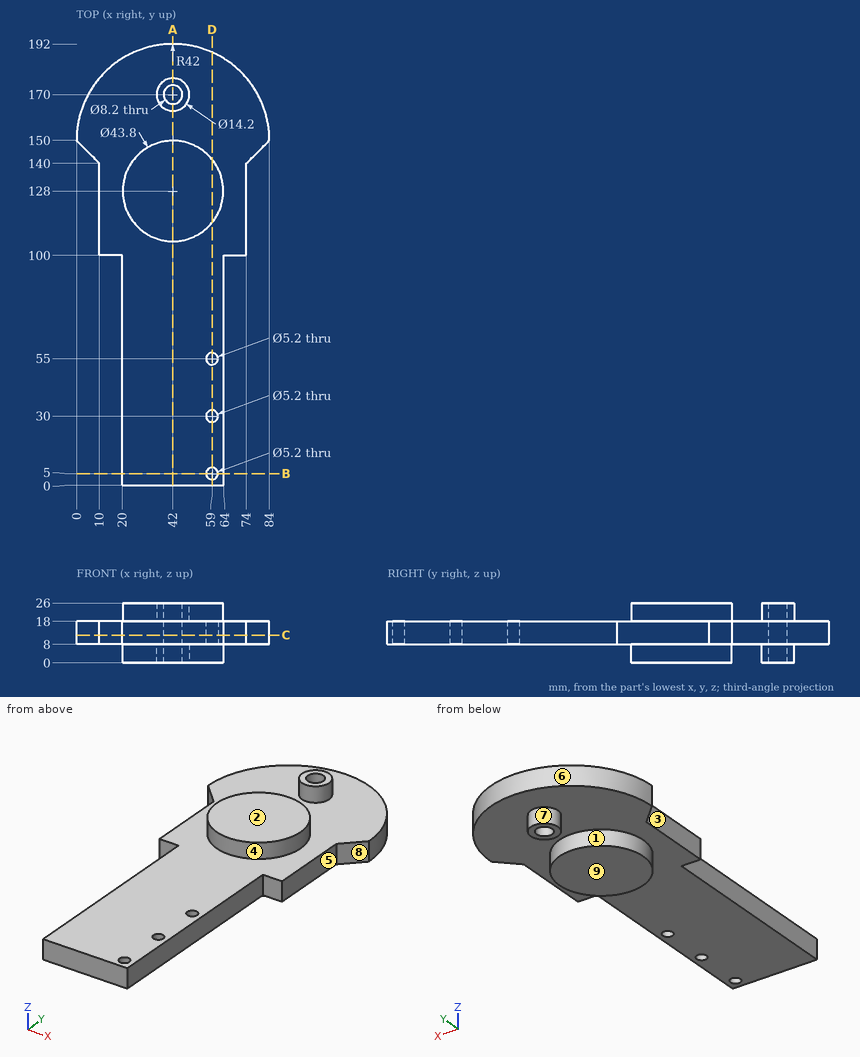
Check sheet for the drawn part. Datum: minimum x, y, z corner. Units: mm. A direction names the side the tool comes from. Round coordinates to 2 decimals unless told otherwise and drop trailing zeros. Order: outer loops, then holes, each group sorted by start corner. A loop starts at its lowest first (then second) coordinate and runs counter-clockwise, first axis right, second up.
(1) Scan lines: probe 1 along Y at (x, z) = (42, 23.5); probe 2 along Y at (x, z) = (42, 11); probe 3 along Y at (x, z) = (59, 12). Record each from-to range of solid material in increasing order.
(2) Cross-section at D-D, the plane x = 59. Enter the section's corners in (y, z), and give its area (3 significant figures).
(3) Access from +Z, -Z, +X, -X, +Y, -Y to the whole of each face (thin tool, end or side, straight path). Record for the marked faces 1, 2, 3, 4 and 5.
(4) Draft check along Y on the marked faces 6, 7, 8 and 9. Enter one of: pulls with the +Y half, pulls with the -Y half, needs draft (parallel to the pull), parting line crosses it, or undercut.
(5) Cross-section at B-B, the plane y = 5. Enter the section's corners in (x, z), and give its area (3 significant figures).
(6) Go/stop test with flat-tipped pins: P1, Ø6, axis at x = 59, y = 30, coming from the +Z side; P2, Ø10, axis at x = 51, y = 35.5, coming from the -Z side; P3, Ø1, axis at y = 172, z = 8.5, coming from the -X side. Record where each tip stops, or that it passes through.
(7) Cross-section at C-C, the plane z = 12. Enter the section's corners in (x, y), and give its area (3 significant figures).
(8) Cross-section at A-A, the plane x = 42. Enter the section's corners in (y, z), and give its area (3 significant figures).
Check sheet entries:
1. probe 1: y = 106.1 to 149.9, 162.9 to 165.9, 174.1 to 177.1
1. probe 2: y = 0 to 165.9, 174.1 to 192
1. probe 3: y = 0 to 2.4, 7.6 to 27.4, 32.6 to 52.4, 57.6 to 188.41
2. outline: (0, 8) - (2.4, 8) - (2.4, 18) - (0, 18) - close; (7.6, 8) - (27.4, 8) - (27.4, 18) - (7.6, 18) - close; (32.6, 8) - (52.4, 8) - (52.4, 18) - (32.6, 18) - close; (57.6, 8) - (114.19, 8) - (114.19, 0) - (141.81, 0) - (141.81, 8) - (188.41, 8) - (188.41, 18) - (141.81, 18) - (141.81, 26) - (114.19, 26) - (114.19, 18) - (57.6, 18) - close
2. area: 2,170 mm2
3. face 1: -Z
3. face 2: +Z, +X, -X, +Y, -Y
3. face 3: +Z, -Z, -X, -Y
3. face 4: +Z
3. face 5: +Z, -Z, +X, -Y
4. face 6: pulls with the +Y half
4. face 7: undercut
4. face 8: pulls with the -Y half
4. face 9: needs draft
5. outline: (20, 8) - (56.4, 8) - (56.4, 18) - (20, 18) - close; (61.6, 8) - (64, 8) - (64, 18) - (61.6, 18) - close
5. area: 388 mm2
6. P1: stops at z = 18
6. P2: stops at z = 8
6. P3: stops at x = 5.92
7. outline: (0, 150) - (10, 140) - (10, 100) - (20, 100) - (20, 0) - (64, 0) - (64, 100) - (74, 100) - (74, 140) - (84, 150) arc R42 ccw to start; hole circle Ø8.2 at (42, 170); hole circle Ø5.2 at (59, 5); hole circle Ø5.2 at (59, 30); hole circle Ø5.2 at (59, 55)
7. area: 10,400 mm2
8. outline: (0, 8) - (106.1, 8) - (106.1, 0) - (149.9, 0) - (149.9, 8) - (162.9, 8) - (162.9, 0) - (165.9, 0) - (165.9, 26) - (162.9, 26) - (162.9, 18) - (149.9, 18) - (149.9, 26) - (106.1, 26) - (106.1, 18) - (0, 18) - close; (174.1, 0) - (177.1, 0) - (177.1, 8) - (192, 8) - (192, 18) - (177.1, 18) - (177.1, 26) - (174.1, 26) - close
8. area: 2,630 mm2
